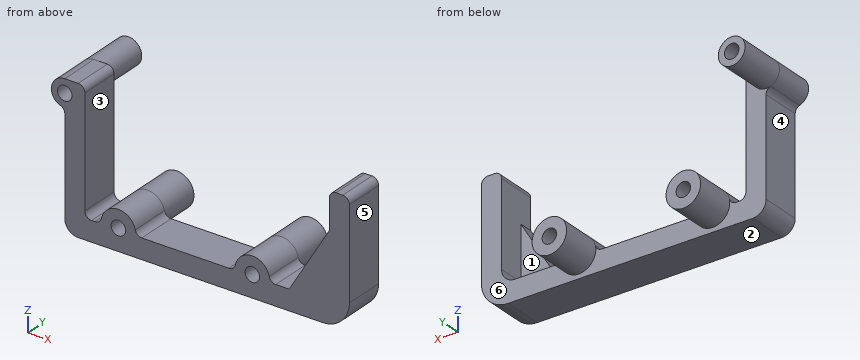
from build123d import *
from build123d.topology import SkipClean

# Parameters (mm, degrees)
SKETCH2_R                      = 3.429
BOSS_EXTRUDE1_DEPTH            = 19.05
SKETCH3_R                      = 8.1915
SKETCH3_R_2                    = 3.429
SKETCH3_R_3                    = 6.35
BOSS_EXTRUDE2_DEPTH            = 19.05
SKETCH4_R                      = 6.35
SKETCH4_R_2                    = 3.429
BOSS_EXTRUDE5_DEPTH            = 3.429
BOSS_EXTRUDE6_START            = -19.05
BOSS_EXTRUDE6_DEPTH            = 6.35
CUT_EXTRUDE2_REACH             = 162.972
SKETCH7_W                      = 141.2875
SKETCH7_H                      = 67.437060646
CUT_EXTRUDE2_DIRECTION_2_REACH = 162.972


with BuildPart() as part:
    # Sketch2 → Boss-Extrude1 (new body)
    with BuildSketch(Plane(origin=(0, 0, 0), x_dir=(1, 0, 0), z_dir=(0, 1, 0))):
        with BuildLine():
            Line((57.144932013, -15.875), (98.430067987, -15.875))
            ThreePointArc((98.430067987, -15.875), (100.422636409, -16.578098691), (101.532702627, -18.375994594))
            ThreePointArc((101.532702627, -18.375994594), (109.5375, -24.828560646), (117.542297372, -18.375994594))
            ThreePointArc((117.542297372, -18.375994594), (118.652363591, -16.578098691), (120.644932013, -15.875))
            Line((120.644932013, -15.875), (122.2375, -15.875))
            ThreePointArc((122.2375, -15.875), (124.48256403, -16.80493597), (125.4125, -19.05))
            Line((125.4125, -19.05), (125.4125, -70.612060646))
            ThreePointArc((125.4125, -70.612060646), (126.34243597, -72.857124676), (128.5875, -73.787060646))
            Line((128.5875, -73.787060646), (134.9375, -73.787060646))
            ThreePointArc((134.9375, -73.787060646), (141.196050854, -68.510858211), (137.054166667, -61.450223232))
            ThreePointArc((137.054166667, -61.450223232), (135.520123355, -60.28989163), (134.9375, -58.456804525))
            Line((134.9375, -58.456804525), (134.9375, -12.7))
            ThreePointArc((134.9375, -12.7), (133.07762806, -8.209871939), (128.5875, -6.35))
            Line((128.5875, -6.35), (12.7, -6.35))
            ThreePointArc((12.7, -6.35), (3.719743879, -10.069743879), (0, -19.05))
            Line((0, -19.05), (0, -61.948583794))
            ThreePointArc((0, -61.948583794), (0.92993597, -64.193647824), (3.175, -65.123583794))
            Line((3.175, -65.123583794), (6.35, -65.123583794))
            ThreePointArc((6.35, -65.123583794), (8.59506403, -64.193647824), (9.525, -61.948583794))
            Line((9.525, -61.948583794), (9.525, -22.225))
            ThreePointArc((9.525, -22.225), (11.384871939, -17.734871939), (15.875, -15.875))
            Line((15.875, -15.875), (34.930067987, -15.875))
            ThreePointArc((34.930067987, -15.875), (36.922636409, -16.578098691), (38.032702627, -18.375994594))
            ThreePointArc((38.032702627, -18.375994594), (46.0375, -24.828560646), (54.042297372, -18.375994594))
            ThreePointArc((54.042297372, -18.375994594), (55.152363591, -16.578098691), (57.144932013, -15.875))
        make_face()
        with Locations(Location((46.0375, -16.637060646, 0), (0, 0, 270))):
            Circle(SKETCH2_R, mode=Mode.SUBTRACT)
        with Locations(Location((109.5375, -16.637060646, 0), (0, 0, 270))):
            Circle(SKETCH2_R, mode=Mode.SUBTRACT)
        with Locations(Location((134.9375, -67.437060646, 0), (0, 0, 270))):
            Circle(SKETCH2_R, mode=Mode.SUBTRACT)
    boss_extrude1 = extrude(amount=-BOSS_EXTRUDE1_DEPTH)

    # Sketch3 → Boss-Extrude2 (add)
    with BuildSketch(Plane(origin=(0, 0, 0), x_dir=(1, 0, 0), z_dir=(0, 1, 0))):
        with Locations(Location((46.0375, -16.637060646, 0), (0, 0, 270))):
            Circle(SKETCH3_R)
        with Locations(Location((46.0375, -16.637060646, 0), (0, 0, 270))):
            Circle(SKETCH3_R_2, mode=Mode.SUBTRACT)
        with Locations(Location((109.5375, -16.637060646, 0), (0, 0, 270))):
            Circle(SKETCH3_R)
        with Locations(Location((109.5375, -16.637060646, 0), (0, 0, 270))):
            Circle(SKETCH3_R_2, mode=Mode.SUBTRACT)
        with Locations(Location((134.9375, -67.437060646, 0), (0, 0, 270))):
            Circle(SKETCH3_R_3)
        with Locations(Location((134.9375, -67.437060646, 0), (0, 0, 270))):
            Circle(SKETCH3_R_2, mode=Mode.SUBTRACT)
    boss_extrude2 = extrude(amount=BOSS_EXTRUDE2_DEPTH)

    # Sketch4 → Boss-Extrude5 (add)
    with BuildSketch(Plane(origin=(0, 19.05, 0), x_dir=(1, 0, 0), z_dir=(0, 1, 0))):
        with Locations(Location((134.9375, -67.437060646, 0), (0, 0, 270))):
            Circle(SKETCH4_R)
        with Locations(Location((134.9375, -67.437060646, 0), (0, 0, 270))):
            Circle(SKETCH4_R_2, mode=Mode.SUBTRACT)
    boss_extrude5 = extrude(amount=BOSS_EXTRUDE5_DEPTH)

    # Sketch6 → Boss-Extrude6 (add)
    with BuildSketch(Plane(origin=(0, 0, 0), x_dir=(1, 0, 0), z_dir=(0, 1, 0)).offset(BOSS_EXTRUDE6_START)):
        Polygon((28.575, -15.875), (9.525, -47.625), (9.525, -15.875), align=None)
    boss_extrude6 = extrude(amount=BOSS_EXTRUDE6_DEPTH)

    # Mirror4: Boss-Extrude1, Boss-Extrude2, Boss-Extrude5, Boss-Extrude6 across plane
    with SkipClean():  # the faces are left unmerged after this step: merging them gives an invalid solid
        add(boss_extrude1.mirror(Plane(origin=(0, -19.05, 19.05), x_dir=(0, 0, 1), z_dir=(-1, 0, 0))))
        add(boss_extrude2.mirror(Plane(origin=(0, -19.05, 19.05), x_dir=(0, 0, 1), z_dir=(-1, 0, 0))))
        add(boss_extrude5.mirror(Plane(origin=(0, -19.05, 19.05), x_dir=(0, 0, 1), z_dir=(-1, 0, 0))))
        add(boss_extrude6.mirror(Plane(origin=(0, -19.05, 19.05), x_dir=(0, 0, 1), z_dir=(-1, 0, 0))))

    # Cut-Extrude2: up to this face of the body (flat: up to its plane)
    cut_extrude2_end = Plane(part.part.faces().sort_by_distance((134.9375, 22.479, 61.266665768))[0])
    # Sketch7 → Cut-Extrude2 (cut, up to the picked face)
    with BuildSketch(Plane(origin=(0, 0, 0), x_dir=(1, 0, 0), z_dir=(0, 1, 0)), mode=Mode.PRIVATE) as cut_extrude2_sk1:
        with Locations((70.64375, -40.068530323)):
            Rectangle(SKETCH7_W, SKETCH7_H)
    cut_extrude2_tool1 = split(extrude(cut_extrude2_sk1.sketch, amount=CUT_EXTRUDE2_REACH, mode=Mode.PRIVATE), bisect_by=cut_extrude2_end, keep=Keep.BOTH, mode=Mode.PRIVATE)
    add(cut_extrude2_tool1.solids().sort_by(Axis((70.64375, 0, 40.06853), (0, 1, 0)))[0], mode=Mode.SUBTRACT)

    # Cut-Extrude2 direction 2: up to this face of the body (flat: up to its plane)
    cut_extrude2_direction_2_end = Plane(part.part.faces().sort_by_distance((0.921292425, -19.05, 25.561080077))[0])
    # Sketch7 → Cut-Extrude2 direction 2 (cut, up to the picked face)
    with BuildSketch(Plane(origin=(0, 0, 0), x_dir=(1, 0, 0), z_dir=(0, 1, 0)), mode=Mode.PRIVATE) as cut_extrude2_direction_2_sk1:
        with Locations((70.64375, -40.068530323)):
            Rectangle(SKETCH7_W, SKETCH7_H)
    cut_extrude2_direction_2_tool1 = split(extrude(cut_extrude2_direction_2_sk1.sketch, amount=-CUT_EXTRUDE2_DIRECTION_2_REACH, mode=Mode.PRIVATE), bisect_by=cut_extrude2_direction_2_end, keep=Keep.BOTH, mode=Mode.PRIVATE)
    add(cut_extrude2_direction_2_tool1.solids().sort_by(Axis((70.64375, 0, 40.06853), (0, -1, 0)))[0], mode=Mode.SUBTRACT)


solid = part.part
Part model, mm, in its own coordinate system. Face numbers are marked on the shaded views. A direction names the side the tool comes from. Give positions to 0.01 mm unless a question says otherwise; leave off trailing zeros. Write each loop counter-clockwise with the first axis right and the second up, starting at its lowest first coordinate (ties: lowest second). Pieces come first, ordered by that corner, then holes.
1) Two-plate mould, pull along X, no slides. Class the marked faces 4, 5 and 6: released by +X, released by -X, zero draft, split by the parting line, or undercut.
Resolved:
face 4: released by -X
face 5: released by +X
face 6: undercut
2) Which spindle directions (+Z, -Z, +X, -X, +Y, -Y) get a long thin tool onto all of the face, cutting with end or side? Do the marked faces 1, 2 and 3. Say none if no direction does.
Resolved:
face 1: +Z, +Y
face 2: -Z, +X, -X, +Y, -Y
face 3: +Z, +Y, -Y
3) Probe L1, parallel to X at y = -15, z = 55 (1 decimal); L2, parallel to X at y = -7.5, z = 21.5; L3, parallel to Z at x = -30, y = -16 (3 decimals). List the from-to ranges inside material, lowest first.
Resolved:
L1: x = -134.9 to -125.4, -9.5 to 0
L2: x = -134.94 to -125.41, -116.13 to -102.95, -52.63 to -39.45, -9.57 to 0
L3: z = 6.35 to 15.875
4) Cut at C-C on x = -27. Write the cut outline in (y, z) (3 decimals), then the cut area to 3 significant figures.
Resolved:
outline: (-19.05, 6.35) - (0, 6.35) - (0, 15.875) - (-12.7, 15.875) - (-12.7, 18.5) - (-19.05, 18.5) - close
area: 198 mm2
5) Cut at D-D on y = -15. State how many separate pieces and enclosed holes the cut face has, then the cut area to 3 significant figures.
Resolved:
separate pieces: 1
enclosed holes: 3
area: 2,760 mm2
6) Cut at B-B on y = 13.5. Write the cut outline in (x, z), then the cut area to 3 significant figures.
Resolved:
outline: circle Ø12.7 at (-134.94, 67.44); circle Ø16.38 at (-109.54, 16.64); circle Ø16.38 at (-46.04, 16.64); hole circle Ø6.86 at (-134.94, 67.44); hole circle Ø6.86 at (-109.54, 16.64); hole circle Ø6.86 at (-46.04, 16.64)
area: 437 mm2
7) Pin check, flat tips, straight feed: pin 1 (12 mm diameter, centred on x = -88.5, y = 7, fed in from -Z); pin 2 (2 mm diameter, centred on x = -76, y = 0, fed in from +Z) (3 decimals); pin 3 (15 mm diameter, centred on x = -29, y = -12.5, fed in from +Z); pin 4 (2 mm diameter, centred on y = -10, z = 45.5, fed in from -X). Stop position of each tip, or through.
Resolved:
pin 1: passes through
pin 2: stops at z = 15.875
pin 3: stops at z = 27.66
pin 4: stops at x = -134.94
